Here's the drawing with two shaded views (mm, measured from the low corner). I have some questions. A direction names the side the tool comes from. Round coordinates to 2 decimals unless told otherwise and drop trailing zeros. Order: outer loops, then holes, each group sorted by start corner. A loop starts at its lowest first (then second) coordinate and runs counter-clockwise, first axis right, second up. Notation, with made-up numbers: M 79,64.25 L 91,64.25 A15 ccw 91,68.25 Z; hole C 69,-18 d2. An arc over 180 degrees is marked long. One line per question, with ' | ' between items.
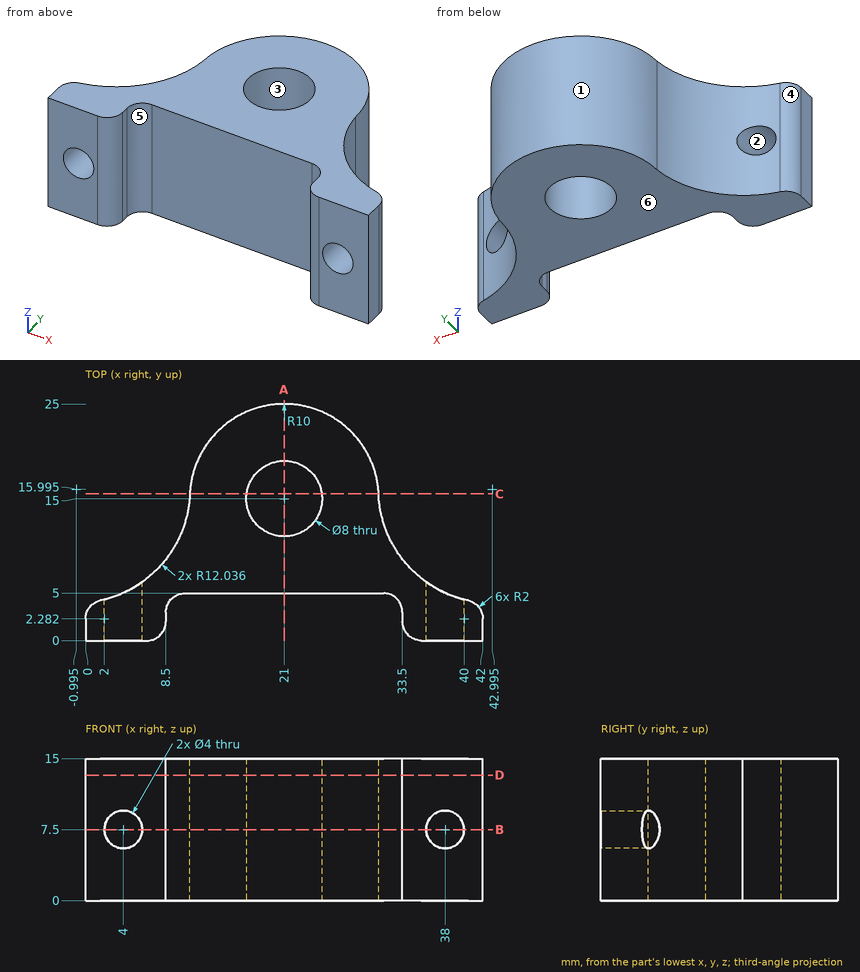
(1) Please list where these lines run through material, in increasing order: probe 1 along X at (y, z) = (2.25, 7.5); probe 2 along Z at (x, y) = (4, 4.5); probe 3 along X at (y, z) = (3.5, 7.5) (1 decimal). Write a range as [from, to].
Final values:
probe 1: [0, 2], [6, 8.5], [33.5, 36], [40, 42] | probe 2: [0, 5.5], [9.5, 15] | probe 3: [0.4, 2], [6, 8.6], [33.4, 36], [40, 41.6]
(2) Will these pins go through, and if not, where does the flat tip stop? pin 1 Ø3 at (y, z) = (16.5, 9) entering from +X; pin 2 Ø8 at (y, z) = (7.5, 8.5) entering from +X; pin 3 Ø3 at (x, z) = (4, 7.5) entering from -Y; pin 4 Ø6 at (x, z) = (25, 2) entering from -Y.
Final values:
pin 1: x = 31 | pin 2: x = 41.59 | pin 3: through | pin 4: y = 5
(3) If we section it at C-C on y = 15.5: Please give me the cut outline in (x, z), plus the area to 3 significant figures.
Final values:
outline: M 11.01,0 L 17.03,0 L 17.03,15 L 11.01,15 Z; M 24.97,0 L 30.99,0 L 30.99,15 L 24.97,15 Z | area: 181 mm^2
(4) If we section it at D-D on z = 13.25: Please give me the cut outline in (x, y) (1 decimal), plus the area to 3 significant figures.
Final values:
outline: M 0,0 L 6.5,0 A2 ccw 8.5,2 L 8.5,3 A2 cw 10.5,5 L 31.5,5 A2 cw 33.5,3 L 33.5,2 A2 ccw 35.5,0 L 42,0 L 42,2.3 A2 ccw 40.4,4.2 A12 cw 31,15 A10 ccw 11,15 A12 cw 1.6,4.2 A2 ccw 0,2.3 Z; hole C 21,15 d8 | area: 429 mm^2
(5) On a 3-axis mill with a long thin cutter (end or side, diameter ignored), from which of +Z, -Z, +X, -X, +Y, -Y can I reach the whole of each face in a straight line? I mean the marked faces 5 and 6. Say none if no direction works.
Final values:
face 5: +Z, -Z, -Y | face 6: -Z, +X, -X, +Y, -Y
(6) If we section it at B-B on z = 7.5: Please give me the cut outline in (x, y) (1 decimal), plus the area to 3 significant figures.
Final values:
outline: M 0,0 L 2,0 L 2,4.3 A12 cw 1.6,4.2 A2 ccw 0,2.3 Z; M 6,0 L 6.5,0 A2 ccw 8.5,2 L 8.5,3 A2 cw 10.5,5 L 31.5,5 A2 cw 33.5,3 L 33.5,2 A2 ccw 35.5,0 L 36,0 L 36,6.2 A12 cw 31,15 A10 ccw 11,15 A12 cw 6,6.2 Z; M 40,0 L 42,0 L 42,2.3 A2 ccw 40.4,4.2 A12 cw 40,4.3 Z; hole C 21,15 d8 | area: 388 mm^2
(7) Thinking about a two-plate mould opening in X: for the marked faces 1, 2, 3 and 4, which applies, released by +X, released by -X, zero draft, split by the parting line, or undercut?
Final values:
face 1: split by the parting line | face 2: undercut | face 3: undercut | face 4: released by -X
(8) If we section it at A-A on x = 21: Please give me the cut outline in (y, z).
Final values:
outline: M 5,0 L 11,0 L 11,15 L 5,15 Z; M 19,0 L 25,0 L 25,15 L 19,15 Z
